```python
from build123d import *

# Parameters (mm, degrees)
F0_W     = 508
F0_H     = 660.4
F1_DEPTH = 914.4
F2_W     = 6.35
F2_H     = 660.4
F3_DEPTH = 431.8
F4_W     = 6.35
F4_H     = 431.8
F5_DEPTH = 501.65


with BuildPart() as f1:
    # F0 (on Top) → F1 (new body)
    with BuildSketch(Plane.XY):
        with Locations((254, -330.2)):
            Rectangle(F0_W, F0_H)
    extrude(amount=F1_DEPTH)

    # F2 (on face) → F3 (join)
    with BuildSketch(Plane.XY.offset(914.4)):
        with Locations((3.175, -330.2)):
            Rectangle(F2_W, F2_H)
    extrude(amount=F3_DEPTH)

    # F4 (on face) → F5 (join)
    with BuildSketch(Plane.YZ.offset(6.35)):
        with Locations((-3.175, 1130.3)):
            Rectangle(F4_W, F4_H)
    extrude(amount=F5_DEPTH)


solid = f1.part
```
CAD build for the part. Positions are in the model's coordinates, mm. A direction names the side the tool comes from. Coordinates: 2 decimals unless noted, no trailing zeros. Order: outer loops, then holes, each group sorted by start corner. A loop starts at its lowest first (then second) coordinate and runs counter-clockwise, first axis right, second up.
(1) Drill centre lines: L1, parallel to Z at x = 394, y = -540.5; L2, parallel to Y at x = 34.5, z = 972; L3, parallel to X at y = -180, z = 1254.5. Where is each one in solid material? Low to high.
Solution:
L1: z = 0 to 914.4
L2: y = -6.35 to 0
L3: x = 0 to 6.35
(2) Pin check, flat tips, straight feed: pin 1 Ø12 at (x, y) = (266, -554.5) entering from -Z; pin 2 Ø2 at (x, y) = (266, -568) entering from +Z. Stop position of each tip, or through.
Solution:
pin 1: stops at z = 0
pin 2: stops at z = 914.4
(3) Saw through at B-B, the plane y = -249. Write the cut outline in (x, z), and give its area (3 significant figures).
Solution:
outline: (0, 0) - (508, 0) - (508, 914.4) - (6.35, 914.4) - (6.35, 1346.2) - (0, 1346.2) - close
area: 467,000 mm2
(4) Which spindle directions (+Z, -Z, +X, -X, +Y, -Y) get a long thin tool onto all of the face, cutting with end or side? Do faces 1 (the face through (250, 0, 664)), 2 (the face through (254, -329, 914.4)). Say none if no direction does.
Solution:
face 1: +Z, -Z, +X, -X, +Y
face 2: +Z, +X, -Y
(5) Saw through at A-A, the plane z = 1082. Write the cut outline in (x, y), and give its area (3 significant figures).
Solution:
outline: (0, -660.4) - (6.35, -660.4) - (6.35, -6.35) - (508, -6.35) - (508, 0) - (0, 0) - close
area: 7,380 mm2
